from build123d import *

# Parameters (mm, degrees)
F2_SIZE  = 0.2
F3_R     = 1.25
F4_DEPTH = 1.501


with BuildPart() as f1:
    # F0 (on Front) → F1 (revolve)
    with BuildSketch(Plane.XZ):
        with BuildLine():
            Line((7.5, -1.5), (9, -1.5))
            Line((9, -1.5), (9, 0))
            ThreePointArc((9, 0), (8.56066, -1.06066), (7.5, -1.5))
        make_face()
        with BuildLine():
            Line((0, -1.5), (7.5, -1.5))
            ThreePointArc((7.5, -1.5), (6.43934, -1.06066), (6, 0))
            Line((6, 0), (0, 0))
            Line((0, 0), (0, -1.5))
        make_face()
        with BuildLine():
            ThreePointArc((6, 0), (6.43934, -1.06066), (7.5, -1.5))
            ThreePointArc((7.5, -1.5), (8.56066, -1.06066), (9, 0))
            ThreePointArc((9, 0), (7.5, 1.5), (6, 0))
        make_face()
    revolve(axis=Axis((0, 0, 0), (0, 0, -1)))

    # F2
    f2_edges = [f1.edges().sort_by_distance(p)[0] for p in [
        (-9, 0, -1.5),
    ]]
    chamfer(f2_edges, length=F2_SIZE)

    # F3 (on face) → F4 (cut, through all)
    with BuildSketch(Plane.XY):
        with Locations((-1.95877, 2.696016)):
            Circle(F3_R)
        with Locations((1.95877, 2.696016)):
            Circle(F3_R)
        with Locations((3.169357, -1.029787)):
            Circle(F3_R)
        with Locations((0, -3.332459)):
            Circle(F3_R)
        with Locations((-3.169357, -1.029787)):
            Circle(F3_R)
    extrude(amount=-F4_DEPTH, mode=Mode.SUBTRACT)


solid = f1.part
For this review, take the finished solid that the model builds, in its own axes (mm). A direction names the side the tool comes from. Coordinates: 2 decimals unless noted, no trailing zeros. Order: outer loops, then holes, each group sorted by start corner. A loop starts at its lowest first (then second) coordinate and runs counter-clockwise, first axis right, second up. Notation, with made-up numbers: (47.25, -7) - (84.25, -7) arc R33 cw to (84.25, 30) - close; hole circle Ø11 at (29, 58). An arc over 180 degrees is marked (long way). Use one line per item in the form item = value.
Q1. Draft analysis for pull direction Y (two halves, no side actions). For faces 3 (the cylindrical face through (-1.172, -8.923, -0.641)), 4 (the cylindrical face through (-0.804, 2.217, -0.74)), 5 (the flat face through (0, 0, -1.5)), 6 (the cylindrical face through (1.92, -0.97, -0.74)), state which applies: +Y half, -Y half, draft (parallel to the pull), parting line (faces both ways), or undercut.
Checked values:
face_3 = parting line
face_4 = undercut
face_5 = draft
face_6 = undercut
Q2. Consider section C-C (z = 1). Give the boundary of the cut face in (x, y).
Checked values:
outline = circle Ø17.24 at (0, 0); hole circle Ø12.76 at (0, 0)
Q3. For P1, Ø3, axis at x = 1.96, y = 2.7, coming from the +Z side; P2, Ø2, axis at x = 3.17, y = -1.03, coming from the +Z side; P3, Ø1.5, axis at y = -3, z = 1, coming from the -X side, all flat-tipped, find the tip position at first contact; note any pin that passes through.
Checked values:
P1 = 0
P2 = through
P3 = -8.58
Q4. For faces 1 (the cylindrical face through (-0.2, -2.1, -0.7)), 2 (the flat face through (0, 0, 0)), list the 3-axis set-ups (+Z, -Z, +X, -X, +Y, -Y) from which the entire face can be reached by the end or side of a thin tool; tool diameter is ignored.
Checked values:
face_1 = +Z, -Z
face_2 = +Z
Q5. Consider section A-A (x = 0). Give the boundary of the cut face in (y, z), then the cut area to 3 significant figures.
Checked values:
outline = (-9, -1.3) - (-8.8, -1.5) - (-4.58, -1.5) - (-4.58, 0) - (-6, 0) arc R1.5 ccw to (-9, 0) - close; (-2.08, -1.5) - (8.8, -1.5) - (9, -1.3) - (9, 0) arc R1.5 ccw to (6, 0) - (-2.08, 0) - close
area = 30.3 mm2
Q6. Consider section D-D (x = 3). Give the number of separate pieces and of enclosed holes in the cut face, then the cut area to 3 significant figures.
Checked values:
separate_pieces = 3
enclosed_holes = 0
area = 27.4 mm2
Q7. Consider section B-B (y = 0). Give the boundary of the cut face in (x, z), then the cut area to 3 significant figures.
Checked values:
outline = (-9, -1.3) - (-8.8, -1.5) - (-3.88, -1.5) - (-3.88, 0) - (-6, 0) arc R1.5 ccw to (-9, 0) - close; (-2.46, -1.5) - (2.46, -1.5) - (2.46, 0) - (-2.46, 0) - close; (3.88, -1.5) - (8.8, -1.5) - (9, -1.3) - (9, 0) arc R1.5 ccw to (6, 0) - (3.88, 0) - close
area = 29.8 mm2
Q8. For probe 1 along Y at (x, z) = (0, -0.9); probe 2 along Y at (x, z) = (2.25, -1.2); probe 3 along X at (y, z) = (2, -0.7), list the stretches that pass through material, from the lowest coordinate up. Write a range as from..to.
Checked values:
probe_1 = -9..-4.58, -2.08..9
probe_2 = -8.71..-1.88, -0.18..1.48, 3.91..8.71
probe_3 = -8.77..-3, -0.92..0.92, 3..8.77
